The model under review builds one solid part; all positions refer to its coordinate system, in mm. A direction names the side the tool comes from. Coordinates: 2 decimals unless noted, no trailing zeros. Write each loop counter-clockwise with the first axis right and the second up, starting at its lowest first coordinate (ties: lowest second). Pieces come first, ordered by that corner, then holes. Notation, with made-up numbers: (62.25, -31.75) - (98.25, -31.75) arc R36 ccw to (98.25, 4.25) - close; hole circle Ø2 at (-23.75, 57). An arc over 180 degrees is marked (long way). Put each result on its own line as item: value.
from build123d import *

# Parameters (mm, degrees)
F1_W     = 10
F1_H     = 34
F1_H_2   = 10
F1_W_2   = 34
F2_DEPTH = 1
F3_ANGLE = 45
F4_W     = 50
F4_H     = 14
F5_DEPTH = 1
F6_R     = 4.99999


# Not quite as in the source:
# - a fillet or chamfer is up to 0.001 mm smaller than in the source, because OpenCascade refuses the exact size


with BuildPart() as f2:
    # F1 (on Top) → F2 (new body)
    with BuildSketch(Plane.XY):
        with Locations((0, -22)):
            Rectangle(F1_W, F1_H)
        Rectangle(F1_W, F1_H_2)
        with Locations((22, 0)):
            Rectangle(F1_W_2, F1_H_2)
        with Locations((-22, 0)):
            Rectangle(F1_W_2, F1_H_2)
        with Locations((0, 22)):
            Rectangle(F1_W, F1_H)
    extrude(amount=F2_DEPTH)


with BuildPart() as f2_1:
    # F3: moved
    add(f2.part.rotate(Axis((0, 0, 15.9228555858), (0, 0, 1)), F3_ANGLE))

    # F4 (on Top) → F5 (join)
    with BuildSketch(Plane.XY):
        Rectangle(F4_W, F4_H)
    extrude(amount=F5_DEPTH)

    # F6 (radius 5 in the source; OpenCascade refuses exactly that, so slightly less here)
    f6_edges = [f2_1.edges().sort_by_distance(p)[0] for p in [
        (-31.112698, 24.041631, 0.5),
        (-31.112698, -24.041631, 0.5),
        (-24.041631, -31.112698, 0.5),
        (24.041631, -31.112698, 0.5),
        (31.112698, 24.041631, 0.5),
        (31.112698, -24.041631, 0.5),
        (24.041631, 31.112698, 0.5),
        (-24.041631, 31.112698, 0.5),
    ]]
    fillet(f6_edges, radius=F6_R)


solid = f2_1.part
1. Consider section C-C on x = -16.5. State the section outline as (y, z) points.
Determined:
outline: (-23.57, 0) - (-9.43, 0) - (-9.43, 1) - (-23.57, 1) - close; (-7, 0) - (7, 0) - (7, 1) - (-7, 1) - close; (9.43, 0) - (23.57, 0) - (23.57, 1) - (9.43, 1) - close
2. Machinability: for faces 1 (the flat face through (-20.73, -13.66, 0.49)), 2 (the flat face through (10.4, 17.47, 0.49)), 3 (the flat face through (20.92, -13.85, 0.49)), 4 (the flat face through (-10.4, -17.47, 0.49)), which of the approach directions +Z, -Z, +X, -X, +Y, -Y give a long, thin tool a straight path to every point of the face, cutting with its end or side? Answer none if there is none.
Determined:
face 1: +Z, -Z, -X
face 2: +Z, -Z, +Y
face 3: +Z, -Z, +X
face 4: +Z, -Z, -Y
3. Consider section D-D on y = -2. State the section outline as (x, z) points, plus the area to 3 significant figures.
Determined:
outline: (-25, 0) - (25, 0) - (25, 1) - (-25, 1) - close
area: 50.0 mm^2
4. To check wall thickness, follow probe 1 along Y at (x, z) = (21.5, 0.65); probe 2 along Y at (x, z) = (-19, 0.35); probe 3 along X at (y, z) = (-10.5, 0.85). State the ranges of each line that lie inside material, in increasing order.
Determined:
probe 1: y = -28.35 to -14.43, -7 to 7, 14.43 to 28.35
probe 2: y = -26.07 to -11.93, -7 to 7, 11.93 to 26.07
probe 3: x = -17.57 to -3.43, 3.43 to 17.57
5. The part is to be moulded in two halves that separate along Y. For faces 5 (the flat face through (-10.11, 17.18, 0.49)), 6 (the flat face through (-20.73, 13.66, 0.49)), 7 (the flat face through (10.11, -17.18, 0.49)), say which applies: +Y half, -Y half, draft (parallel to the pull), parting line (faces both ways), or undercut.
Determined:
face 5: +Y half
face 6: undercut
face 7: -Y half
6. For pin 1 Ø0.5 at (x, z) = (18.5, 0.5) entering from -Y, flat-tipped, find the tip position at first contact; note if it passes through.
Determined:
pin 1: stops at y = -25.82
7. Consider section A-A on y = -25. State the section outline as (x, z) points.
Determined:
outline: (-28.95, 0) - (-17.93, 0) - (-17.93, 1) - (-28.95, 1) - close; (17.93, 0) - (28.95, 0) - (28.95, 1) - (17.93, 1) - close
